The listing builds one solid part. Answer for the finished solid, in the listing's coordinates (mm). Face numbers are marked on the shaded views. A direction names the side the tool comes from. Give positions to 0.01 mm unless a question says otherwise; leave off trailing zeros. Order: outer loops, then holes, each group sorted by start corner. A loop starts at its lowest first (then second) coordinate and runs counter-clockwise, first axis right, second up.
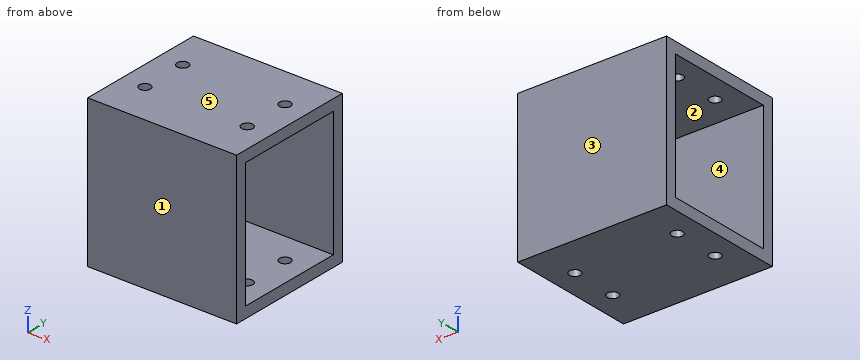
```python
from build123d import *

# Parameters (mm, degrees)
F0_W     = 70
F0_H     = 80
F0_W_2   = 58
F0_H_2   = 68
F1_DEPTH = 80
F3_D     = 6


with BuildPart() as f1:
    # F0 (on Right) → F1 (new body)
    with BuildSketch(Plane.YZ):
        with Locations((-35, 40)):
            Rectangle(F0_W, F0_H)
        with Locations((-35, 40)):
            Rectangle(F0_W_2, F0_H_2, mode=Mode.SUBTRACT)
    extrude(amount=F1_DEPTH)

    # F3 (through all)
    with Locations(Plane.XY.offset(80)):
        with Locations((12.5, -22.5), (67.5, -22.5), (67.5, -47.5), (12.5, -47.5)):
            Hole(F3_D / 2)


solid = f1.part
```
1) Find section D-D (x = 67.5). Write down the section's boundary in (y, z), then the cut area to 3 significant figures.
Geometry says:
outline: (-70, 0) - (-50.5, 0) - (-50.5, 6) - (-64, 6) - (-64, 74) - (-50.5, 74) - (-50.5, 80) - (-70, 80) - close; (-44.5, 0) - (-25.5, 0) - (-25.5, 6) - (-44.5, 6) - close; (-44.5, 74) - (-25.5, 74) - (-25.5, 80) - (-44.5, 80) - close; (-19.5, 0) - (0, 0) - (0, 80) - (-19.5, 80) - (-19.5, 74) - (-6, 74) - (-6, 6) - (-19.5, 6) - close
area: 1,510 mm2
2) For a pull along Y with two mould halves and no side action, classify the marked faces 1, 2 and 3 as +Y half, -Y half, draft (parallel to the pull), parting line (faces both ways), or undercut.
Geometry says:
face 1: -Y half
face 2: undercut
face 3: +Y half
3) Find section A-A (z = 31.5). Write down the section's boundary in (x, y), then the cut area to 3 significant figures.
Geometry says:
outline: (0, -70) - (80, -70) - (80, -64) - (0, -64) - close; (0, -6) - (80, -6) - (80, 0) - (0, 0) - close
area: 960 mm2
4) A tool of negligible diameter and unlimited length cuts with its end or side. For the marked faces 4 and 5, from which of +Z, -Z, +X, -X, +Y, -Y can it reach the whole face along a straight path? Write none if from no direction.
Geometry says:
face 4: +X, -X
face 5: +Z, +X, -X, +Y, -Y
5) Find section B-B (y = -47.5). Write down the section's boundary in (x, z), then the cut area to 3 significant figures.
Geometry says:
outline: (0, 0) - (9.5, 0) - (9.5, 6) - (0, 6) - close; (0, 74) - (9.5, 74) - (9.5, 80) - (0, 80) - close; (15.5, 0) - (64.5, 0) - (64.5, 6) - (15.5, 6) - close; (15.5, 74) - (64.5, 74) - (64.5, 80) - (15.5, 80) - close; (70.5, 0) - (80, 0) - (80, 6) - (70.5, 6) - close; (70.5, 74) - (80, 74) - (80, 80) - (70.5, 80) - close
area: 816 mm2
6) Given P1, Ø3.5, axis at x = 12.5, y = -47.5, coming from the +Z side, flat-ended and moving along its own axis, determine where the tip first touches the part or whether it passes through.
Geometry says:
P1: passes through
7) Find section C-C (x = 17). Write down the section's boundary in (y, z).
Geometry says:
outline: (-70, 0) - (0, 0) - (0, 80) - (-70, 80) - close; hole (-64, 6) - (-6, 6) - (-6, 74) - (-64, 74) - close
8) Straight lines are drawn through the part: probe 1 along Y at (x, z) = (67.5, 78.1); probe 2 along Z at (x, y) = (24, -13); probe 3 along Y at (x, z) = (42, 8.5). For each, find the intervals that lie inside material, in ascending order.
Geometry says:
probe 1: y = -70 to -50.5, -44.5 to -25.5, -19.5 to 0
probe 2: z = 0 to 6, 74 to 80
probe 3: y = -70 to -64, -6 to 0
